from build123d import *

# Parameters (mm, degrees)
EXTRUDE_THIN1_DEPTH = 12.7
SKETCH2_R           = 4.1656
CUT_EXTRUDE1_DEPTH  = 4.175
SKETCH3_R           = 3.2639
CUT_EXTRUDE2_DEPTH  = 4.175
FILLET1_R           = 1.5875


with BuildPart() as part:
    # Sketch1 → Extrude-Thin1 (new body, symmetric)
    with BuildSketch(Plane(origin=(0, 0, 0), x_dir=(0, 0, -1), z_dir=(1, 0, 0))):
        Polygon((25.4, 0), (0, 0), (0, 25.4), (3.175, 25.4), (3.175, 3.175), (25.4, 3.175), align=None)
    extrude(amount=EXTRUDE_THIN1_DEPTH, both=True)

    # Sketch2 → Cut-Extrude1 (cut, through all)
    with BuildSketch(Plane(origin=(0, 0, -3.175), x_dir=(-1, 0, 0), z_dir=(0, 0, -1))):
        with Locations((0, 12.7)):
            Circle(SKETCH2_R)
    extrude(amount=-CUT_EXTRUDE1_DEPTH, mode=Mode.SUBTRACT)

    # Sketch3 → Cut-Extrude2 (cut, through all)
    with BuildSketch(Plane(origin=(0, 3.175, 0), x_dir=(1, 0, 0), z_dir=(0, 1, 0))):
        with Locations(Location((0, 12.7, 0), (0, 0, 270))):  # turned: the seam where the file's is
            Circle(SKETCH3_R)
    extrude(amount=-CUT_EXTRUDE2_DEPTH, mode=Mode.SUBTRACT)

    # Fillet1
    fillet1_edges = [part.edges().sort_by_distance(p)[0] for p in [
        (0, 25.4, -3.175),
        (0, 3.175, -3.175),
        (0, 3.175, -25.4),
    ]]
    fillet(fillet1_edges, radius=FILLET1_R)


solid = part.part
Design review of the part built by this model. Coordinates are the model's own, in mm. A direction names the side the tool comes from. Give positions to 0.01 mm unless a question says otherwise; leave off trailing zeros. Write each loop counter-clockwise with the first axis right and the second up, starting at its lowest first coordinate (ties: lowest second). Pieces come first, ordered by that corner, then holes. Notation, with made-up numbers: M 58,7.25 L 93,7.25 A28 ccw 93,36.25 Z; hole C -38,47.25 d10. An arc over 180 degrees is marked long. Return JSON: item names as keys, results as strings. Group by question number.
Item 1: Take a section at D-D (x = 6.75). Give the boundary of the cut face in (y, z) (1 decimal), plus the area to 3 significant figures.
Item 2: Clearance check with flat-ended pins moving along their axes: pin 1 Ø5.5 at (x, y) = (5.5, 13.5) entering from -Z (3 decimals); pin 2 Ø5.5 at (x, z) = (1, -15) entering from +Y (3 decimals). State where each tip first meets the part, or that it passes through.
Item 3: Tool access review of faces 5 (the cylindrical face through (-1.986, 1.61, -15.29)), 6 (the flat face through (0.2, 3.175, -16.3)): name each direction out of +Z, -Z, +X, -X, +Y, -Y from which nothing blocks a thin tool from reaching the whole face with its end or side.
Item 4: The part is to be moulded in two halves that separate along Y. For faces 1 (the flat face through (3, 0, -10)), 2 (the flat face through (0, 25.4, -1)), 3 (the cylindrical face through (0.54, 16.83, -1.61)), 4 (the flat face through (3, 17, -3.175)), say which applies: pulls with the +Y half, pulls with the -Y half, needs draft (parallel to the pull), parting line crosses it, or undercut.
Item 5: Wall thickness on line 1 along X through (y, z) = (2.45, -12.7); line 2 along Y through (x, z) = (6.25, -11.75) (3 decimals); line 3 along Z through (x, y) = (8.25, 9) (3 decimals): over which ranges is each line inside the solid? List them lowest first.
Item 6: Take a section at C-C (z = -12.25). Give the boundary of the cut face in (x, y) (3 decimals), plus the area to 3 significant figures.
Item 7: Take a section at A-A (x = 0). Give the boundary of the cut face in (y, z) (1 decimal).
Item 8: Take a section at B-B (y = 12.7). Give the boundary of the cut face in (x, z) (3 decimals), plus the area to 3 significant figures.
Return value:
{
 "1": {"outline": "M 0,-25.4 L 1.6,-25.4 A1.6 ccw 3.2,-23.8 L 3.2,-4.8 A1.6 cw 4.8,-3.2 L 23.8,-3.2 A1.6 ccw 25.4,-1.6 L 25.4,0 L 0,0 Z", "area": "151 mm2"},
 "2": {"pin 1": "stops at z = -3.175", "pin 2": "stops at y = 3.175"},
 "3": {"face 5": "+Y, -Y", "face 6": "-Z, +X, -X, +Y"},
 "4": {"face 1": "pulls with the -Y half", "face 2": "pulls with the +Y half", "face 3": "undercut", "face 4": "needs draft"},
 "5": {"line 1": "x = -12.7 to -3.26, 3.26 to 12.7", "line 2": "y = 0 to 3.175", "line 3": "z = -3.175 to 0"},
 "6": {"outline": "M -12.7,0 L -3.233,0 L -3.233,3.175 L -12.7,3.175 Z; M 3.233,0 L 12.7,0 L 12.7,3.175 L 3.233,3.175 Z", "area": "60.1 mm2"},
 "7": {"outline": "M 0,-25.4 L 1.6,-25.4 A1.6 ccw 3.2,-23.8 L 3.2,-16 L 0,-16 Z; M 0,-9.4 L 3.2,-9.4 L 3.2,-4.8 A1.6 cw 4.8,-3.2 L 8.5,-3.2 L 8.5,0 L 0,0 Z; M 16.9,-3.2 L 23.8,-3.2 A1.6 ccw 25.4,-1.6 L 25.4,0 L 16.9,0 Z"},
 "8": {"outline": "M -12.7,-3.175 L -4.166,-3.175 L -4.166,0 L -12.7,0 Z; M 4.166,-3.175 L 12.7,-3.175 L 12.7,0 L 4.166,0 Z", "area": "54.2 mm2"}
}
